Geometry check sheet. Reference: the model listing, model coordinates, mm. A direction names the side the tool comes from. Round coordinates to 2 decimals unless told otherwise and drop trailing zeros. Order: outer loops, then holes, each group sorted by start corner. A loop starts at its lowest first (then second) coordinate and runs counter-clockwise, first axis right, second up. Notation, with made-up numbers: (25, 80) - (77, 80) arc R24 cw to (77, 90) - close; hole circle Ø11 at (50, -19.75). An arc over 180 degrees is marked (long way). One line per question, with ' | ' between items. Start each with the question number.
Q1. Sectioned sample at C-C, the plane z = -18. Enter the section's corners in (x, y) (1 decimal).
Q2. Material ranges on line 1 along Z through (x, y) = (0, -2.3); line 2 along Z through (x, y) = (2.5, 1.25); line 3 along Z through (x, y) = (-2.5, -2), recorded low to high.
Q3. Mould release check, pull along X, two halves, no side actions. Record for faces 4 (the face through (0, 3.175, 1)), 5 (the face through (-3.112, -2.1, -12.2)), 6 (the face through (3.112, -2.1, -12.2)), 7 (the face through (-0.12, -2.18, -30.26)): +X half, -X half, draft (parallel to the pull), parting line (faces both ways), or undercut.
Q4. Tool access check on faces 1 (the face through (0, 2.032, 2)), 2 (the face through (0, -1.905, -16)), 3 (the face through (0, -3, -32.322)). Record the directions out of +Z, -Z, +X, -X, +Y, -Y that give a thin tool (end or side, any length) a straight path to the whole face; none if there is none.
Q5. Sectioned sample at D-D, the plane y = 0.75. Enter the section's corners in (x, z).
Q6. Sectioned sample at B-B, the plane x = -2. Enter the section's corners in (y, z) (1 decimal), then the cut area to 3 significant figures.
Q7. Sectioned sample at A-A, the plane x = 0. Enter the section's corners in (y, z) (1 decimal), then the cut area to 3 significant figures.
Q8. Gauge pin test, flat ends, axial feed: P1, Ø1.6, axis at x = 0, y = -2, coming from the +Z side; P2, Ø2.5, axis at x = 0, z = -29.38, coming from the +Y side (3 decimals). Record the tip position at first contact, or that the pin passes through.
```python
from build123d import *

# Parameters (mm, degrees)
SKETCH1_W                                      = 6.223
SKETCH1_H                                      = 1.143
BOSS_EXTRUDE1_DEPTH                            = 3.175
SKETCH2_W                                      = 6.223
SKETCH2_H                                      = 1.143
BOSS_EXTRUDE2_DEPTH                            = 2.032
SKETCH3_W                                      = 6.223
SKETCH3_H                                      = 1.27
BOSS_EXTRUDE3_DEPTH                            = 31.75
CSK_FOR_0_FLAT_HEAD_MACHINE_SCREW1_D           = 1.778
CSK_FOR_0_FLAT_HEAD_MACHINE_SCREW1_DEPTH       = 4.572
CSK_FOR_0_FLAT_HEAD_MACHINE_SCREW1_CSINK_D     = 3.0226
CSK_FOR_0_FLAT_HEAD_MACHINE_SCREW1_CSINK_ANGLE = 82
CSK_FOR_0_FLAT_HEAD_MACHINE_SCREW1_TIP         = 0.53416509


with BuildPart() as part:
    # Sketch1 → Boss-Extrude1 (new, symmetric)
    with BuildSketch(Plane(origin=(0, 0, 0), x_dir=(1, 0, 0), z_dir=(0, 1, 0))):
        Rectangle(SKETCH1_W, SKETCH1_H)
    extrude(amount=BOSS_EXTRUDE1_DEPTH, both=True)

    # Sketch2 → Boss-Extrude2 (add)
    with BuildSketch(Plane.XY.offset(0.5715)):
        with Locations((0, 2.6035)):
            Rectangle(SKETCH2_W, SKETCH2_H)
    extrude(amount=BOSS_EXTRUDE2_DEPTH)

    # Sketch3 → Boss-Extrude3 (add)
    with BuildSketch(Plane(origin=(0, 0, -0.5715), x_dir=(-1, 0, 0), z_dir=(0, 0, -1))):
        with Locations((0, -2.54)):
            Rectangle(SKETCH3_W, SKETCH3_H)
    extrude(amount=BOSS_EXTRUDE3_DEPTH)

    # CSK for #0 Flat Head Machine Screw1
    with Locations(Plane(origin=(0, -3.175, 0), x_dir=(-1, 0, 0), z_dir=(0, -1, 0))):
        with Locations((0, 29.378038883)):
            CounterSinkHole(CSK_FOR_0_FLAT_HEAD_MACHINE_SCREW1_D / 2, CSK_FOR_0_FLAT_HEAD_MACHINE_SCREW1_CSINK_D / 2, depth=CSK_FOR_0_FLAT_HEAD_MACHINE_SCREW1_DEPTH, counter_sink_angle=CSK_FOR_0_FLAT_HEAD_MACHINE_SCREW1_CSINK_ANGLE)
            with Locations((0, 0, -(CSK_FOR_0_FLAT_HEAD_MACHINE_SCREW1_DEPTH + CSK_FOR_0_FLAT_HEAD_MACHINE_SCREW1_TIP / 2))):  # 118° drill point
                Cone(0, CSK_FOR_0_FLAT_HEAD_MACHINE_SCREW1_D / 2, CSK_FOR_0_FLAT_HEAD_MACHINE_SCREW1_TIP, mode=Mode.SUBTRACT)


solid = part.part
```
Determined:
1) outline: (-3.1, -3.2) - (3.1, -3.2) - (3.1, -1.9) - (-3.1, -1.9) - close
2) line 1: z = -32.32 to -30.27, -28.49 to 0.57 | line 2: z = -0.57 to 0.57 | line 3: z = -32.32 to 0.57
3) face 4: draft | face 5: -X half | face 6: +X half | face 7: undercut
4) face 1: +Z, +X, -X, -Y | face 2: -Z, +X, -X, +Y | face 3: -Z, +X, -X, +Y, -Y
5) outline: (-3.11, -0.57) - (3.11, -0.57) - (3.11, 0.57) - (-3.11, 0.57) - close
6) outline: (-3.2, -32.3) - (-1.9, -32.3) - (-1.9, -0.6) - (3.2, -0.6) - (3.2, 2.6) - (2, 2.6) - (2, 0.6) - (-3.2, 0.6) - close | area: 49.9 mm2
7) outline: (-3.2, -32.3) - (-1.9, -32.3) - (-1.9, -30.3) - (-2.5, -30.3) - (-3.2, -30.9) - close; (-3.2, -27.9) - (-2.5, -28.5) - (-1.9, -28.5) - (-1.9, -0.6) - (3.2, -0.6) - (3.2, 2.6) - (2, 2.6) - (2, 0.6) - (-3.2, 0.6) - close | area: 47.2 mm2
8) P1: stops at z = 0.57 | P2: stops at y = -1.905
